Can you work these out from the model? Positions are in its coordinate system, mm. A direction names the side the tool comes from. Give positions to 0.01 mm unless a question says otherwise; leave off trailing zeros. Write each loop counter-clockwise with the first axis right and the second up, starting at its lowest first coordinate (ties: lowest second). Pieces come first, ordered by that corner, then holes.
```python
from build123d import *

# Parameters (mm, degrees)
SKETCH8_W             = 20
SKETCH8_H             = 20
BOSS_EXTRUDE5_DEPTH   = 600
BOSS_EXTRUDE5_2_DEPTH = 600
SKETCH10_W            = 900
SKETCH10_H            = 600
SKETCH10_W_2          = 860
SKETCH10_H_2          = 560
BOSS_EXTRUDE6_DEPTH   = 20
SKETCH12_W            = 900
SKETCH12_H            = 600
SKETCH12_W_2          = 860
SKETCH12_H_2          = 560
BOSS_EXTRUDE7_DEPTH   = 20
SKETCH13_W            = 20
SKETCH13_H            = 560
BOSS_EXTRUDE8_DEPTH   = 20
SKETCH14_W            = 20
SKETCH14_H            = 20
BOSS_EXTRUDE9_DEPTH   = 350
SKETCH16_W            = 900
SKETCH16_H            = 600
SKETCH16_W_2          = 860
SKETCH16_H_2          = 560
BOSS_EXTRUDE10_DEPTH  = 20
SKETCH17_W            = 200
SKETCH17_H            = 620
CUT_EXTRUDE1_DEPTH    = 601
SKETCH18_W            = 20
SKETCH18_H            = 20
BOSS_EXTRUDE11_DEPTH  = 620
SKETCH19_W            = 20
SKETCH19_H            = 20
BOSS_EXTRUDE12_DEPTH  = 560


with BuildPart() as part:
    # Sketch8 → Boss-Extrude5 (new body)
    with BuildSketch(Plane(origin=(0, 0, 4.872076023), x_dir=(-1, 0, 0), z_dir=(0, 0, -1))):
        with Locations((-1040, 690)):
            Rectangle(SKETCH8_W, SKETCH8_H)
    extrude(amount=BOSS_EXTRUDE5_DEPTH)



with BuildPart() as body_2:
    # Sketch8 → Boss-Extrude5 2 (new body)
    with BuildSketch(Plane(origin=(0, 0, 4.872076023), x_dir=(-1, 0, 0), z_dir=(0, 0, -1))):
        with Locations((-1040, 110)):
            Rectangle(SKETCH8_W, SKETCH8_H)
    extrude(amount=BOSS_EXTRUDE5_2_DEPTH)


with BuildPart() as part_1:
    add(part.part)

    add(body_2.part)  # Boss-Extrude6 merges body 2
    # Sketch10 → Boss-Extrude6 (add)
    with BuildSketch(Plane(origin=(0, 0, -595.127923977), x_dir=(-1, 0, 0), z_dir=(0, 0, -1))):
        with Locations((-600, 400)):
            Rectangle(SKETCH10_W, SKETCH10_H)
        with Locations((-600, 400)):
            Rectangle(SKETCH10_W_2, SKETCH10_H_2, mode=Mode.SUBTRACT)
    extrude(amount=BOSS_EXTRUDE6_DEPTH)

    # Sketch12 → Boss-Extrude7 (add)
    with BuildSketch(Plane.XY.offset(-245.127923977)):
        with Locations((600, 400)):
            Rectangle(SKETCH12_W, SKETCH12_H)
        with Locations((600, 400)):
            Rectangle(SKETCH12_W_2, SKETCH12_H_2, mode=Mode.SUBTRACT)
    extrude(amount=BOSS_EXTRUDE7_DEPTH)

    # Sketch13 → Boss-Extrude8 (add)
    with BuildSketch(Plane(origin=(0, 0, -615.127923977), x_dir=(-1, 0, 0), z_dir=(0, 0, -1))):
        with Locations((-360, 400)):
            Rectangle(SKETCH13_W, SKETCH13_H)
    boss_extrude8 = extrude(amount=-BOSS_EXTRUDE8_DEPTH)

    # Mirror1: Boss-Extrude8 across plane
    add(boss_extrude8.mirror(Plane(origin=(0, 0, -420.127923977), x_dir=(1, 0, 0), z_dir=(0, 0, -1))))

    # Sketch14 → Boss-Extrude9 (add)
    with BuildSketch(Plane(origin=(0, 0, -245.127923977), x_dir=(-1, 0, 0), z_dir=(0, 0, -1))):
        with Locations((-360, 610)):
            Rectangle(SKETCH14_W, SKETCH14_H)
    boss_extrude9 = extrude(amount=BOSS_EXTRUDE9_DEPTH)

    # Mirror2: Boss-Extrude9 across plane
    add(boss_extrude9.mirror(Plane(origin=(0, 560, 0), x_dir=(0, 0, 1), z_dir=(0, -1, 0))))

    # Sketch16 → Boss-Extrude10 (add)
    with BuildSketch(Plane.XY.offset(-85.127923977)):
        with Locations((600, 400)):
            Rectangle(SKETCH16_W, SKETCH16_H)
        with Locations((600, 400)):
            Rectangle(SKETCH16_W_2, SKETCH16_H_2, mode=Mode.SUBTRACT)
    extrude(amount=BOSS_EXTRUDE10_DEPTH)

    # Sketch17 → Cut-Extrude1 (cut, through all)
    with BuildSketch(Plane(origin=(0, 700, 0), x_dir=(1, 0, 0), z_dir=(0, 1, 0))):
        with Locations((250, 305.127923977)):
            Rectangle(SKETCH17_W, SKETCH17_H)
    extrude(amount=-CUT_EXTRUDE1_DEPTH, mode=Mode.SUBTRACT)

    # Sketch18 → Boss-Extrude11 (add)
    with BuildSketch(Plane(origin=(0, 0, -615.127923977), x_dir=(-1, 0, 0), z_dir=(0, 0, -1))):
        with Locations((-360, 690)):
            Rectangle(SKETCH18_W, SKETCH18_H)
        with Locations((-360, 110)):
            Rectangle(SKETCH18_W, SKETCH18_H)
    extrude(amount=-BOSS_EXTRUDE11_DEPTH)

    # Sketch19 → Boss-Extrude12 (add)
    with BuildSketch(Plane.XZ.offset(-680)):
        with Locations((360, -75.127923977)):
            Rectangle(SKETCH19_W, SKETCH19_H)
    extrude(amount=BOSS_EXTRUDE12_DEPTH)


solid = part_1.part
```
1) For faces 3 (the face through (1030, 690, -30)), 4 (the face through (360, 680, -156)), 5 (the face through (1040, 120, -30)), 6 (the face through (370, 690, -423)), 7 (the face through (705, 120, -605)), which set-ups out of +Z, -Z, +X, -X, +Y, -Y let a thin tool reach every point of the face, with its end or its side?
Values follow:
face 3: +Z, +Y, -Y
face 4: +X, -X
face 5: +Z, +X, -X
face 6: +Y, -Y
face 7: +Z, -Z
2) For pin 1 Ø6 at (x, y) = (667, 114.5) entering from +Z, with a flat end and sliding along its axis, tell me the tip position at first contact or that it passes through.
Values follow:
pin 1: stops at z = -65.13
3) Suppose I cut it at C-C on z = -185. Write out the boundary of the cut face in (x, y), plus the area to 3 significant figures.
Values follow:
outline: (350, 100) - (370, 100) - (370, 120) - (350, 120) - close; (350, 680) - (370, 680) - (370, 700) - (350, 700) - close; (1030, 100) - (1050, 100) - (1050, 120) - (1030, 120) - close; (1030, 680) - (1050, 680) - (1050, 700) - (1030, 700) - close
area: 1,600 mm2
4) Suppose I cut it at B-B on z = -408. Write out the boundary of the cut face in (x, y), plus the area to 3 significant figures.
Values follow:
outline: (350, 100) - (370, 100) - (370, 120) - (350, 120) - close; (350, 500) - (370, 500) - (370, 520) - (350, 520) - close; (350, 600) - (370, 600) - (370, 620) - (350, 620) - close; (350, 680) - (370, 680) - (370, 700) - (350, 700) - close; (1030, 100) - (1050, 100) - (1050, 120) - (1030, 120) - close; (1030, 680) - (1050, 680) - (1050, 700) - (1030, 700) - close
area: 2,400 mm2
5) Suppose I cut it at A-A on y = 221. Write out the boundary of the cut face in (x, z).
Values follow:
outline: (350, -615.13) - (370, -615.13) - (370, -595.13) - (350, -595.13) - close; (350, -245.13) - (370, -245.13) - (370, -225.13) - (350, -225.13) - close; (350, -85.13) - (370, -85.13) - (370, -65.13) - (350, -65.13) - close; (1030, -615.13) - (1050, -615.13) - (1050, -595.13) - (1030, -595.13) - close; (1030, -245.13) - (1050, -245.13) - (1050, -225.13) - (1030, -225.13) - close; (1030, -85.13) - (1050, -85.13) - (1050, -65.13) - (1030, -65.13) - close
6) Please list where these lines run through material, in increasing order: L1, parallel to Y at x = 503.5, z = -80; L2, parallel to X at y = 516.5, z = -356.
Values follow:
L1: y = 100 to 120, 680 to 700
L2: x = 350 to 370
7) If we mould it in two halves opening along X, with no side actions, what happens to faces 1 (the face through (360, 404, -225.128)), 2 (the face through (695, 690, -65.128))? For each: +X half, -X half, draft (parallel to the pull), parting line (faces both ways), or undercut.
Values follow:
face 1: draft
face 2: undercut
